Can you work these out from the model? Positions are in its coordinate system, mm. Face numbers are marked on the shaded views. A direction names the side the tool comes from. Give positions to 0.01 mm unless a question says otherwise; leave off trailing zeros. Write each loop counter-clockwise with the first axis right and the second up, starting at its lowest first coordinate (ties: lowest second). Pieces come first, ordered by that corner, then holes. Notation, with made-up numbers: (28, 25.25) -> (43, 25.25) arc R17 ccw to (43, 53.25) -> close; hole circle Ø3 at (52, 67.5). An arc over 180 degrees is marked (long way). Answer as CSV lines item,"result". Start each with the question number.
1. On a 3-axis mill with a long thin cutter (end or side, diameter ignored), from which of +Z, -Z, +X, -X, +Y, -Y can I reach the whole of each face in a straight line? I mean the marked faces 1 and 2. Say none if no direction works.
2. If we mould it in two halves opening along X, with no side actions, what happens to the marked faces 3 and 4? For each: pulls with the +X half, pulls with the -X half, needs draft (parallel to the pull), parting line crosses it, or undercut.
3. If we section it at D-D on y = 23.5: Write out the boundary of the cut face in (x, z), plus the area to 3 significant figures.
4. If we section it at C-C on x = 27: Write out the boundary of the cut face in (y, z), plus the area to 3 significant figures.
5. I'm going to push flat-ended pins straight in: P1, Ø4, axis at x = 33.5, y = 33, coming from the +Z side; P2, Ø3.5, axis at x = 2.5, y = 32.5, coming from the +Z side; P3, Ø1.6, axis at x = 11.5, z = 2, coming from the -Y side. Where does each tip first touch, or does it pass through?
6. If we section it at A-A on y = 40.64: Count the separate pieces of the cut face and the enclosed holes in it, plus the area to 3 significant figures.
7. I need wall thicknesses on line 1 (X direction, y = 40.64, z = 0.65); line 2 (Y direction, x = 11, z = 2.15). Which ranges of each line are inside material? Lowest first, please. Write a range as [from, to].
8. If we section it at B-B on x = 40.64: Write out the boundary of the cut face in (y, z).
Autodesk Inventor part; units mm, degrees
ref_plane "Work Plane1" through (0, 44.704, 0) normal (0, 1, 0) x (1, 0, 0)
ref_plane "YZ Plane" through (0, 0, 0) normal (1, 0, 0) x (0, 1, 0)
ref_plane "XZ Plane" through (0, 0, 0) normal (0, 1, 0) x (-1, 0, 0)
sketch "Sketch1" plane through (0, 0, 0) normal (0, 0, 1) x (1, 0, 0)
  line L0 (0, 0) -> (43.18, 0)
  line L1 (43.18, 0) -> (43.18, 43.18)
  line L2 (43.18, 43.18) -> (0, 43.18)
  line L3 (0, 43.18) -> (0, 0)
  dimension "d0" = 43.18
  dimension "d1" = 43.18
extrude "Extrusion1" add sketch "Sketch1" along normal blind 0.762
sketch "Sketch2" plane through (0, 0, 0.762) normal (0, 0, 1) x (1, 0, 0)
  line L0 (0, 0) -> (43.18, 0)
  line L1 (43.18, 0) -> (43.18, 43.18)
  line L2 (43.18, 43.18) -> (0, 43.18)
  line L3 (0, 43.18) -> (0, 0)
  line L4 (2.54, 40.64) -> (40.64, 40.64)
  line L5 (40.64, 40.64) -> (40.64, 2.54)
  line L6 (40.64, 2.54) -> (2.54, 2.54)
  line L7 (2.54, 2.54) -> (2.54, 40.64)
  dimension "d4" = 2.54
hole "Hole1" at (2.54, 40.64, 0.762) at (2.54, 2.54, 0.762) at (40.64, 2.54, 0.762) at (40.64, 40.64, 0.762) direction (0, 0, -1) diameter 3.3528 depth 25.4 tip angle 118
ref_plane "Work Plane1" through (0, 44.704, 0) normal (0, 1, 0) x (1, 0, 0)
sketch "Sketch3" plane through (0, 44.704, 0) normal (0, 1, 0) x (1, 0, 0)
  line L0 (43.18, -0.762) -> (0, -0.762)
  line L1 (9.4488, -0.762) -> (15.9512, -0.762)
  line L2 (17.2212, -2.032) -> (17.2212, -2.7432)
  line L3 (15.9512, -4.0132) -> (9.4488, -4.0132)
  line L4 (8.1788, -2.7432) -> (8.1788, -2.032)
  line L5 (0, 0) -> (0, -0.762)
  arc A0 (9.4488, -0.762) -> (8.1788, -2.032) centre (9.4488, -2.032) ccw
  arc A1 (17.2212, -2.032) -> (15.9512, -0.762) centre (15.9512, -2.032) ccw
  arc A2 (15.9512, -4.0132) -> (17.2212, -2.7432) centre (15.9512, -2.7432) ccw
  arc A3 (8.1788, -2.7432) -> (9.4488, -4.0132) centre (9.4488, -2.7432) ccw
  line L6 (0, -0.762) -> (43.18, -0.762)
  line L7 (12.827, -0.762) -> (12.827, 2.5763)
  line L8 (12.7, -4.0132) -> (12.7, -2.4751)
  point P0 (8.1788, -0.762)
  point P1 (17.2212, -4.0132)
  point P2 (17.2212, -0.762)
  point P3 (8.1788, -4.0132)
  dimension "d13" = 9.0424
  dimension "d14" = 3.2512
  dimension "d15" = 8.1788
  dimension "d16" = 1.27
extrude "Extrusion2" add sketch "Sketch3" against normal blind 7.366
sketch "Sketch4" plane through (0, 44.704, 0) normal (0, 1, 0) x (1, 0, 0)
  line L0 (9.4488, -0.762) -> (15.9512, -0.762)
  arc A0 (9.4488, -0.762) -> (8.1788, -2.032) centre (9.4488, -2.032) ccw
  line L1 (8.1788, -2.7432) -> (8.1788, -2.032)
  arc A1 (8.1788, -2.7432) -> (9.4488, -4.0132) centre (9.4488, -2.7432) ccw
  line L2 (15.9512, -4.0132) -> (9.4488, -4.0132)
  arc A2 (15.9512, -4.0132) -> (17.2212, -2.7432) centre (15.9512, -2.7432) ccw
  line L3 (17.2212, -2.032) -> (17.2212, -2.7432)
  arc A3 (17.2212, -2.032) -> (15.9512, -0.762) centre (15.9512, -2.032) ccw
  line L4 (9.4488, -2.032) -> (15.9512, -2.032)
  line L5 (15.9512, -2.032) -> (15.9512, -2.7432)
  line L6 (15.9512, -2.7432) -> (9.4488, -2.7432)
  line L7 (9.4488, -2.7432) -> (9.4488, -2.032)
  arc A4 (9.4488, -0.8459) -> (8.2627, -2.032) centre (9.4488, -2.032) ccw
  line L8 (9.4488, -0.8459) -> (15.9512, -0.8459)
  arc A5 (17.1373, -2.032) -> (15.9512, -0.8459) centre (15.9512, -2.032) ccw
  line L9 (17.1373, -2.032) -> (17.1373, -2.7432)
  arc A6 (15.9512, -3.9293) -> (17.1373, -2.7432) centre (15.9512, -2.7432) ccw
  line L10 (15.9512, -3.9293) -> (9.4488, -3.9293)
  arc A7 (8.2627, -2.7432) -> (9.4488, -3.9293) centre (9.4488, -2.7432) ccw
  line L11 (8.2627, -2.7432) -> (8.2627, -2.032)
  point P0 (0, 0)
extrude "Extrusion3" cut sketch "Sketch4" against normal blind 5.08 contours L8 A5 L9 A6 L10 A7 L11 A4
sketch "Sketch5" plane through (0, 0, 0.762) normal (0, 0, 1) x (1, 0, 0)
  line L0 (9.4488, 43.18) -> (9.4488, 37.338)
  line L1 (9.4488, 43.18) -> (0, 43.18)
  line L2 (0, 43.18) -> (0, 0)
  line L3 (0, 0) -> (43.18, 0)
  line L4 (43.18, 0) -> (43.18, 43.18)
  line L5 (43.18, 43.18) -> (15.9512, 43.18)
  line L6 (15.9512, 43.18) -> (15.9512, 37.338)
  line L7 (15.9512, 37.338) -> (9.4488, 37.338)
  circle A0 centre (40.64, 2.54) radius 1.6764
  circle A1 centre (2.54, 40.64) radius 1.6764
  circle A2 centre (2.54, 2.54) radius 1.6764
  circle A3 centre (40.64, 40.64) radius 1.6764
  line L8 (0, 0) -> (43.18, 0)
  line L9 (21.59, 0) -> (21.59, 11.5828)
  line L10 (0.254, 35.6558) -> (4.4958, 35.6558)
  line L11 (4.4958, 35.6558) -> (4.4958, 29.6868)
  line L12 (4.4958, 29.6868) -> (0.254, 29.6868)
  line L13 (0.254, 29.6868) -> (0.254, 35.6558)
  line L14 (42.926, 35.6558) -> (38.6842, 35.6558)
  line L15 (38.6842, 35.6558) -> (38.6842, 29.6868)
  line L16 (38.6842, 29.6868) -> (42.926, 29.6868)
  line L17 (42.926, 29.6868) -> (42.926, 35.6558)
  dimension "d21" = 4.2418
  dimension "d22" = 5.969
  dimension "d23" = 0.254
extrude "Extrusion4" add sketch "Sketch5" along normal blind 3.0734 contours L10 L11 L12 L13 | L17 L16 L15 L14
sketch "Sketch6" plane through (0, 0, 0.762) normal (0, 0, 1) x (1, 0, 0)
  circle A0 centre (8.128, 4.064) radius 3.1877
  line L0 (0, 43.18) -> (0, 0)
  line L1 (0, 0) -> (43.18, 0)
  line L2 (6.526, 1.3081) -> (9.73, 1.3081)
  line L3 (8.128, 7.2517) -> (14.0521, 7.2517)
  dimension "d26" = 6.3754
  dimension "d27" = 8.128
  dimension "d28" = 4.064
  dimension "d29" = 5.9436
extrude "Extrusion5" cut sketch "Sketch6" against normal through all contours A0 L2 picked at (8.128, 3.2893)
sketch "Sketch7" plane through (0, 0, 0.762) normal (0, 0, 1) x (1, 0, 0)
  line L0 (10.7696, 26.289) -> (32.7406, 26.289)
  line L1 (32.7406, 26.289) -> (32.7406, 9.271)
  line L2 (32.7406, 9.271) -> (10.7696, 9.271)
  line L3 (10.7696, 9.271) -> (10.7696, 26.289)
  line L4 (0, 0) -> (43.18, 0)
  line L5 (0, 43.18) -> (0, 0)
  dimension "d32" = 21.971
  dimension "d33" = 17.018
  dimension "d34" = 9.271
  dimension "d35" = 10.7696
extrude "Extrusion6" add sketch "Sketch7" along normal blind 2.5908
sketch "Sketch8" plane through (0, 0, 0.762) normal (0, 0, 1) x (1, 0, 0)
  circle A0 centre (32.004, 30.1752) radius 3.3782
  line L0 (43.18, 43.18) -> (15.9512, 43.18)
  line L1 (43.18, 0) -> (43.18, 43.18)
  point P0 (0, 0)
  dimension "d38" = 6.7564
  dimension "d39" = 13.0048
  dimension "d40" = 11.176
extrude "Extrusion7" add sketch "Sketch8" along normal blind 2.5908
sketch "Sketch9" plane through (0, 0, 0.762) normal (0, 0, 1) x (1, 0, 0)
  circle A0 centre (15.748, 5.334) radius 0.9906
  circle A1 centre (15.748, 5.334) radius 0.8567
  circle A2 centre (15.748, 5.334) radius 0.3208
  line L0 (0, 43.18) -> (0, 0)
  line L1 (0, 0) -> (43.18, 0)
  dimension "d43" = 1.9812
  dimension "d44" = 15.748
  dimension "d45" = 5.334
extrude "Extrusion8" add sketch "Sketch9" along normal blind 1.27
sketch "Sketch10" plane through (9.4488, 44.704, 4.0132) normal (0, 0, 1) x (1, 0, 0)
  line L0 (-9.4517, -1.8915) -> (33.7316, -1.8915) construction
  line L1 (33.7316, -1.8915) -> (33.7316, -44.7034) construction
  line L2 (33.7316, -44.7034) -> (-9.4517, -44.7034) construction
  line L3 (-9.4517, -44.7034) -> (-9.4517, -1.8915) construction
  point P0 (-9.4488, -44.704)
decal "Decal1"
sketch "Sketch11" plane through (0, 0, 3.3528) normal (0, 0, 1) x (1, 0, 0)
  line L0 (0.004, 42.7411) -> (43.1873, 42.7411) construction
  line L1 (43.1873, 42.7411) -> (43.1873, -0.0708) construction
  line L2 (43.1873, -0.0708) -> (0.004, -0.0708) construction
  line L3 (0.004, -0.0708) -> (0.004, 42.7411) construction
  point P0 (0, 0)
  point P1 (-9.4488, -44.704)
decal "Decal2"
properties part number "SparkFun GPS-RTK2 Board - ZED-F9P"
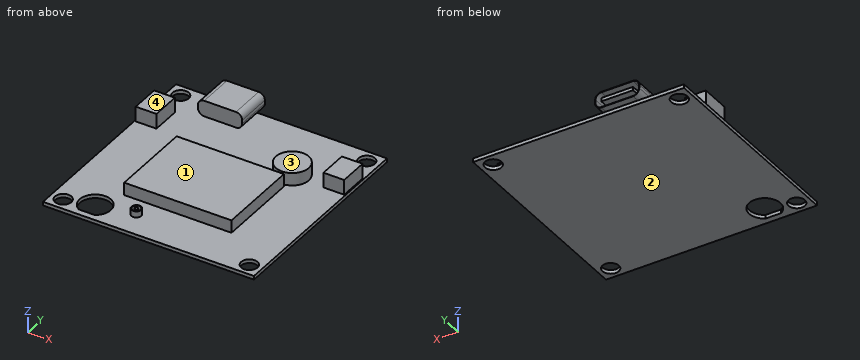
Computed values:
1,face 1,"+Z, +X, -X, -Y"
1,face 2,"-Z, +X, -X, +Y, -Y"
2,face 3,"undercut"
2,face 4,"needs draft"
3,outline,"(0, 0) -> (43.18, 0) -> (43.18, 0.76) -> (32.74, 0.76) -> (32.74, 3.35) -> (10.77, 3.35) -> (10.77, 0.76) -> (0, 0.76) -> close"
3,area,"89.8 mm2"
4,outline,"(0, 0) -> (43.18, 0) -> (43.18, 0.76) -> (26.29, 0.76) -> (26.29, 3.35) -> (9.27, 3.35) -> (9.27, 0.76) -> (0, 0.76) -> close"
4,area,"77.0 mm2"
5,P1,"stops at z = 3.35"
5,P2,"stops at z = 3.84"
5,P3,"stops at y = 9.27"
6,separate pieces,"4"
6,enclosed holes,"1"
6,area,"34.3 mm2"
7,line 1,"x = [0, 0.86], [4.22, 38.96], [42.32, 43.18]"
7,line 2,"y = [9.27, 26.29], [37.34, 44.7]"
8,outline,"(0, 0) -> (0.86, 0) -> (0.86, 0.76) -> (0, 0.76) -> close; (4.22, 0) -> (38.96, 0) -> (38.96, 0.76) -> (35.66, 0.76) -> (35.66, 3.84) -> (29.69, 3.84) -> (29.69, 0.76) -> (4.22, 0.76) -> close; (42.32, 0) -> (43.18, 0) -> (43.18, 0.76) -> (42.32, 0.76) -> close"
